```python
from build123d import *

# Parameters (mm, degrees)
SKETCH1_W           = 4
SKETCH1_H           = 70
SKETCH1_H_2         = 60
BOSS_EXTRUDE1_DEPTH = 3
SKETCH1_3_W         = 4
SKETCH1_3_H         = 60
SKETCH1_3_H_2       = 70
BOSS_EXTRUDE2_DEPTH = 70
SKETCH1_4_W         = 4
SKETCH1_4_H         = 70
BOSS_EXTRUDE3_DEPTH = 70
SKETCH5_R           = 4
CUT_EXTRUDE4_DEPTH  = 10
SKETCH6_R           = 2.5
CUT_EXTRUDE5_DEPTH  = 10
SKETCH1_5_W         = 4
SKETCH1_5_H         = 60
BOSS_EXTRUDE4_DEPTH = 80
SKETCH5_2_R         = 4
CUT_EXTRUDE6_DEPTH  = 10
FILLET1_R           = 3
FILLET2_R           = 5
FILLET3_R           = 4
SKETCH7_R           = 2.5
CUT_EXTRUDE7_DEPTH  = 10
SKETCH8_R           = 2.5
CUT_EXTRUDE8_DEPTH  = 10
CUT_EXTRUDE9_REACH  = 132.084
SKETCH9_R           = 3.5
SKETCH26_R          = 2.5
CUT_EXTRUDE11_DEPTH = 10
CUT_EXTRUDE14_DEPTH = 10
CUT_EXTRUDE15_DEPTH = 10
SKETCH28_R          = 1
SKETCH28_R_2        = 4
CUT_EXTRUDE16_DEPTH = 4
SKETCH29_R          = 1
SKETCH29_R_2        = 3.5
CUT_EXTRUDE18_DEPTH = 4
SKETCH31_R          = 5.375
CUT_EXTRUDE19_DEPTH = 10
SKETCH32_W          = 71.641660037
SKETCH32_H          = 79.51751689
CUT_EXTRUDE20_DEPTH = 131.084107183
SKETCH33_W          = 4
SKETCH33_H          = 70
SKETCH33_H_2        = 60
CUT_EXTRUDE21_DEPTH = 71.771465692


with BuildPart() as part:
    # Sketch1 → Boss-Extrude1 (new body)
    # profile 1 of 4: a face of its own
    with BuildSketch(Plane(origin=(0, 0, 0), x_dir=(1, 0, 0), z_dir=(0, 1, 0))):
        Polygon((-50.771305032, 49.212548619), (-50.771305032, 34.212548619), (-46.771305032, 34.212548619), (-46.771305032, -25.787451381), (-50.771305032, -25.787451381), (-50.771305032, -40.787451381), (39.228694968, -40.787451381), (39.228694968, -30.787451381), (35.228694968, -30.787451381), (35.228694968, 39.212548619), (39.228694968, 39.212548619), (39.228694968, 49.212548619), align=None)
        with Locations((-26.271305032, 3.893815937)):
            Rectangle(SKETCH1_W, SKETCH1_H, mode=Mode.SUBTRACT)
    # profile 2 of 4: a face of its own
    with BuildSketch(Plane(origin=(0, 0, 0), x_dir=(1, 0, 0), z_dir=(0, 1, 0))):
        with Locations((37.228694968, 4.212548619)):
            Rectangle(SKETCH1_W, SKETCH1_H)
    # profile 3 of 4: a face of its own
    with BuildSketch(Plane(origin=(0, 0, 0), x_dir=(1, 0, 0), z_dir=(0, 1, 0))):
        with Locations((-48.771305032, 4.212548619)):
            Rectangle(SKETCH1_W, SKETCH1_H_2)
    # profile 4 of 4: a face of its own
    with BuildSketch(Plane(origin=(0, 0, 0), x_dir=(1, 0, 0), z_dir=(0, 1, 0))):
        with Locations((-26.271305032, 3.893815937)):
            Rectangle(SKETCH1_W, SKETCH1_H)
    extrude(amount=BOSS_EXTRUDE1_DEPTH)

    # Sketch1<3> → Boss-Extrude2 (add)
    with BuildSketch(Plane(origin=(0, 0, 0), x_dir=(1, 0, 0), z_dir=(0, 1, 0))):
        with Locations((-48.771305032, 4.212548619)):
            Rectangle(SKETCH1_3_W, SKETCH1_3_H)
        with Locations((37.228694968, 4.212548619)):
            Rectangle(SKETCH1_3_W, SKETCH1_3_H_2)
    extrude(amount=BOSS_EXTRUDE2_DEPTH)

    # Sketch1<4> → Boss-Extrude3 (add)
    with BuildSketch(Plane(origin=(0, 0, 0), x_dir=(1, 0, 0), z_dir=(0, 1, 0))):
        with Locations((-26.271305032, 3.893815937)):
            Rectangle(SKETCH1_4_W, SKETCH1_4_H)
    extrude(amount=BOSS_EXTRUDE3_DEPTH)

    # Sketch5 → Cut-Extrude4 (cut)
    with BuildSketch(Plane.ZY.offset(50.771305032)):
        with Locations((-8.022548619, 60)):
            Circle(SKETCH5_R)
    extrude(amount=-CUT_EXTRUDE4_DEPTH, mode=Mode.SUBTRACT)

    # Sketch6 → Cut-Extrude5 (cut)
    with BuildSketch(Plane(origin=(0, 3, 0), x_dir=(1, 0, 0), z_dir=(0, 1, 0))):
        with Locations(Location((-45.787574368, -35.787451381, 0), (0, 0, 270))):
            Circle(SKETCH6_R)
        with Locations(Location((-45.787574368, 44.212548619, 0), (0, 0, 270))):
            Circle(SKETCH6_R)
        with Locations((43.718511914, 44.212548619)):
            Circle(SKETCH6_R)
        with Locations((43.718511914, -35.787451381)):
            Circle(SKETCH6_R)
    extrude(amount=-CUT_EXTRUDE5_DEPTH, mode=Mode.SUBTRACT)

    # Sketch1<5> → Boss-Extrude4 (add)
    with BuildSketch(Plane(origin=(0, 0, 0), x_dir=(1, 0, 0), z_dir=(0, 1, 0))):
        with Locations((-48.771305032, 4.212548619)):
            Rectangle(SKETCH1_5_W, SKETCH1_5_H)
    extrude(amount=BOSS_EXTRUDE4_DEPTH)

    # Sketch5<2> → Cut-Extrude6 (cut)
    with BuildSketch(Plane.ZY.offset(50.771305032)):
        with Locations((-8.022548619, 60)):
            Circle(SKETCH5_2_R)
    extrude(amount=-CUT_EXTRUDE6_DEPTH, mode=Mode.SUBTRACT)

    # Fillet1
    fillet1_edges = [part.edges().sort_by_distance(p)[0] for p in [
        (-50.771305032, 1.5, 40.787451381),
        (-50.771305032, 1.5, -49.212548619),
        (39.228694968, 1.5, -49.212548619),
        (39.228694968, 1.5, 40.787451381),
    ]]
    fillet(fillet1_edges, radius=FILLET1_R)

    # Fillet2
    fillet2_edges = [part.edges().sort_by_distance(p)[0] for p in [
        (-48.771305032, 80, -34.212548619),
        (-48.771305032, 80, 25.787451381),
        (37.228694968, 70, -39.212548619),
        (37.228694968, 70, 30.787451381),
    ]]
    fillet(fillet2_edges, radius=FILLET2_R)

    # Fillet3
    fillet3_edges = [part.edges().sort_by_distance(p)[0] for p in [
        (-26.271305032, 70, 31.106184063),
        (-26.271305032, 70, -38.893815937),
    ]]
    fillet(fillet3_edges, radius=FILLET3_R)

    # Sketch7 → Cut-Extrude7 (cut)
    with BuildSketch(Plane(origin=(39.228694968, 0, 0), x_dir=(0, 0, -1), z_dir=(1, 0, 0))):
        with Locations((27.482306935, -10)):
            Circle(SKETCH7_R)
    extrude(amount=-CUT_EXTRUDE7_DEPTH, mode=Mode.SUBTRACT)

    # Sketch8 → Cut-Extrude8 (cut)
    with BuildSketch(Plane(origin=(39.228694968, 0, 0), x_dir=(0, 0, -1), z_dir=(1, 0, 0))):
        with Locations((8.02072759, 38.893893193)):
            Circle(SKETCH8_R)
    extrude(amount=-CUT_EXTRUDE8_DEPTH, mode=Mode.SUBTRACT)

    # Cut-Extrude9: up to this face of the body (flat: up to its plane)
    cut_extrude9_end = Plane(part.part.faces().sort_by_distance((-28.271305032, 36.452186393, -3.893815937))[0])
    # Sketch9 → Cut-Extrude9 (cut, up to the picked face)
    with BuildSketch(Plane(origin=(39.228694968, 0, 0), x_dir=(0, 0, -1), z_dir=(1, 0, 0)), mode=Mode.PRIVATE) as cut_extrude9_sk1:
        with Locations((8.02072759, 38.893893193)):
            Circle(SKETCH9_R)
    cut_extrude9_tool1 = split(extrude(cut_extrude9_sk1.sketch, amount=-CUT_EXTRUDE9_REACH, mode=Mode.PRIVATE), bisect_by=cut_extrude9_end, keep=Keep.BOTH, mode=Mode.PRIVATE)
    add(cut_extrude9_tool1.solids().sort_by(Axis((39.228695, 38.893893, -8.020728), (-1, 0, 0)))[0], mode=Mode.SUBTRACT)

    # Sketch26 → Cut-Extrude11 (cut)
    with BuildSketch(Plane(origin=(0, 3, 0), x_dir=(1, 0, 0), z_dir=(0, 1, 0))):
        with Locations(Location((34.228694968, -36.063353705, 0), (0, 0, 270))):
            Circle(SKETCH26_R)
        with Locations(Location((34.228694968, 44.212548619, 0), (0, 0, 270))):
            Circle(SKETCH26_R)
    extrude(amount=-CUT_EXTRUDE11_DEPTH, mode=Mode.SUBTRACT)

    # Sketch27 → Cut-Extrude14 (cut)
    with BuildSketch(Plane(origin=(0, 3, 0), x_dir=(1, 0, 0), z_dir=(0, 1, 0))):
        with BuildLine():
            Line((7.728694968, 3.462548619), (-19.271305032, 3.462548619))
            ThreePointArc((-19.271305032, 3.462548619), (-20.021305032, 4.212548619), (-19.271305032, 4.962548619))
            Line((-19.271305032, 4.962548619), (7.728694968, 4.962548619))
            ThreePointArc((7.728694968, 4.962548619), (8.478694968, 4.212548619), (7.728694968, 3.462548619))
        make_face()
        with BuildLine():
            Line((0.329175915, -7.853794332), (-13.170824085, 15.52889157))
            ThreePointArc((-13.170824085, 15.52889157), (-12.896305032, 16.553410623), (-11.871785979, 16.27889157))
            Line((-11.871785979, 16.27889157), (1.628214021, -7.103794332))
            ThreePointArc((1.628214021, -7.103794332), (1.353694968, -8.128313385), (0.329175915, -7.853794332))
        make_face()
        with BuildLine():
            Line((-13.170824085, -7.103794332), (0.329175915, 16.27889157))
            ThreePointArc((0.329175915, 16.27889157), (1.353694968, 16.553410623), (1.628214021, 15.52889157))
            Line((1.628214021, 15.52889157), (-11.871785979, -7.853794332))
            ThreePointArc((-11.871785979, -7.853794332), (-12.896305032, -8.128313385), (-13.170824085, -7.103794332))
        make_face()
    extrude(amount=-CUT_EXTRUDE14_DEPTH, mode=Mode.SUBTRACT)

    # Sketch27<7> → Cut-Extrude15 (cut)
    with BuildSketch(Plane(origin=(0, 3, 0), x_dir=(1, 0, 0), z_dir=(0, 1, 0))):
        with BuildLine():
            Line((-7.743699741, 2.296260771), (-7.070343138, 3.462548619))
            Line((-7.070343138, 3.462548619), (-8.417056343, 3.462548619))
            ThreePointArc((-8.417056343, 3.462548619), (-8.152874893, 2.837548619), (-7.743699741, 2.296260771))
        make_face()
        with BuildLine():
            Line((-8.417056343, 4.962548619), (-7.070343138, 4.962548619))
            Line((-7.070343138, 4.962548619), (-7.743699741, 6.128836466))
            ThreePointArc((-7.743699741, 6.128836466), (-8.152874893, 5.587548619), (-8.417056343, 4.962548619))
        make_face()
        with BuildLine():
            Line((-5.771305032, 5.712548619), (-5.09794843, 6.878836466))
            ThreePointArc((-5.09794843, 6.878836466), (-5.771305032, 6.962548619), (-6.444661635, 6.878836466))
            Line((-6.444661635, 6.878836466), (-5.771305032, 5.712548619))
        make_face()
        with BuildLine():
            Line((-4.472266927, 4.962548619), (-3.125553721, 4.962548619))
            ThreePointArc((-3.125553721, 4.962548619), (-3.389735172, 5.587548619), (-3.798910324, 6.128836466))
            Line((-3.798910324, 6.128836466), (-4.472266927, 4.962548619))
        make_face()
        with BuildLine():
            ThreePointArc((-3.798910324, 2.296260771), (-3.389735172, 2.837548619), (-3.125553721, 3.462548619))
            Line((-3.125553721, 3.462548619), (-4.472266927, 3.462548619))
            Line((-4.472266927, 3.462548619), (-3.798910324, 2.296260771))
        make_face()
        with BuildLine():
            ThreePointArc((-6.444661635, 1.546260771), (-5.771305032, 1.462548619), (-5.09794843, 1.546260771))
            Line((-5.09794843, 1.546260771), (-5.771305032, 2.712548619))
            Line((-5.771305032, 2.712548619), (-6.444661635, 1.546260771))
        make_face()
    extrude(amount=-CUT_EXTRUDE15_DEPTH, mode=Mode.SUBTRACT)

    # Sketch28 → Cut-Extrude16 (cut)
    # profile 1 of 3: a face of its own
    with BuildSketch(Plane.ZY.offset(50.771305032)):
        with Locations((-2.316893756, 66.434710762)):
            Circle(SKETCH28_R)
    # profile 2 of 3: a face of its own
    with BuildSketch(Plane.ZY.offset(50.771305032)):
        with Locations((-20.69441, 45.708956331)):
            Circle(SKETCH28_R)
    # profile 3 of 3: a face of its own
    with BuildSketch(Plane.ZY.offset(50.771305032)):
        Polygon((-23.458777666, 51.635023443), (-8.531192269, 68.470022529), (0.44747391, 60.508643651), (-14.480111487, 43.673644564), align=None)
        with Locations((-8.022548619, 60)):
            Circle(SKETCH28_R_2, mode=Mode.SUBTRACT)
    extrude(amount=-CUT_EXTRUDE16_DEPTH, mode=Mode.SUBTRACT)

    # Sketch29 → Cut-Extrude18 (cut)
    # profile 1 of 3: a face of its own
    with BuildSketch(Plane(origin=(39.228694968, 0, 0), x_dir=(0, 0, -1), z_dir=(1, 0, 0))):
        with Locations((2.315072727, 45.328603955)):
            Circle(SKETCH29_R)
    # profile 2 of 3: a face of its own
    with BuildSketch(Plane(origin=(39.228694968, 0, 0), x_dir=(0, 0, -1), z_dir=(1, 0, 0))):
        with Locations((20.692588971, 24.602849525)):
            Circle(SKETCH29_R)
    # profile 3 of 3: a face of its own
    with BuildSketch(Plane(origin=(39.228694968, 0, 0), x_dir=(0, 0, -1), z_dir=(1, 0, 0))):
        Polygon((8.529371241, 47.363915722), (23.456956637, 30.528916636), (14.478290458, 22.567537758), (-0.449294939, 39.402536844), align=None)
        with Locations((8.02072759, 38.893893193)):
            Circle(SKETCH29_R_2, mode=Mode.SUBTRACT)
    extrude(amount=-CUT_EXTRUDE18_DEPTH, mode=Mode.SUBTRACT)

    # Sketch31 → Cut-Extrude19 (cut)
    with BuildSketch(Plane(origin=(0, 3, 0), x_dir=(1, 0, 0), z_dir=(0, 1, 0))):
        with Locations((-5.771305032, 4.212548619)):
            Circle(SKETCH31_R)
    extrude(amount=-CUT_EXTRUDE19_DEPTH, mode=Mode.SUBTRACT)

    # Sketch32 → Cut-Extrude20 (cut, through all)
    with BuildSketch(Plane(origin=(39.228694968, 0, 0), x_dir=(0, 0, -1), z_dir=(1, 0, 0))):
        with Locations((4.714645955, 42.758758445)):
            Rectangle(SKETCH32_W, SKETCH32_H)
    extrude(amount=-CUT_EXTRUDE20_DEPTH, mode=Mode.SUBTRACT)

    # Sketch33 → Cut-Extrude21 (cut, through all)
    with BuildSketch(Plane(origin=(0, 3, 0), x_dir=(1, 0, 0), z_dir=(0, 1, 0))):
        with Locations((-26.271305032, 3.893815937)):
            Rectangle(SKETCH33_W, SKETCH33_H)
        with Locations((-48.771305032, 4.212548619)):
            Rectangle(SKETCH33_W, SKETCH33_H_2)
        with Locations((37.228694968, 4.212548619)):
            Rectangle(SKETCH33_W, SKETCH33_H)
    extrude(amount=-CUT_EXTRUDE21_DEPTH, mode=Mode.SUBTRACT)


solid = part.part
```
Geometry: final body of the model. Coordinates: model frame, mm. A direction names the side the tool comes from. Coordinates: 2 decimals unless noted, no trailing zeros. Order: outer loops, then holes, each group sorted by start corner. A loop starts at its lowest first (then second) coordinate and runs counter-clockwise, first axis right, second up. Notation, with made-up numbers: (-27, 6) - (-18, 6) arc R20 cw to (-18, 10) - close; hole circle Ø4 at (36.25, 80). An arc over 180 degrees is marked (long way). Return JSON: item names as keys, results as strings. Group by question number.
1. Cut plane A-A (z = 13). Output: boundary loops of the cut face in (x, y).
2. Pin query (flat end, axial travel): pin 1 (1.5 mm diameter, centred on x = -49.5, y = 1, fed in from -Z); pin 2 (1.5 mm diameter, centred on y = 1, z = -16.5, fed in from +X); pin 3 (3 mm diameter, centred on x = -25.5, z = -7.5, fed in from -Y). Return the tip coordinate at first contact, or that it passes through.
3. Pull-direction query (Z, two-part tool) for faces 4 (the face through (-6, 1, 40.787)), 5 (the face through (-46.745, 1.521, 38.097)), 6 (the face through (39.229, 1, 34)); classes: pulls with the +Z half, pulls with the -Z half, needs draft (parallel to the pull), parting line crosses it, or undercut.
4. Cut plane B-B (y = 2.3). Count the separate pieces of the cut face and the enclosed holes in it, plus the area to 3 significant figures.
5. Material intervals for line 1 along X through (y, z) = (1, -34); line 2 along Z through (x, y) = (6, 1.7); line 3 along X through (y, z) = (1.1, 27.5), sorted ascending. Write a range as [from, to].
6. Set-up query: faces 1 (the face through (-15, 2, -3.463)), 2 (the face through (-49, 2, -34.213)), 3 (the face through (37, 2, 30.787)). Return all of +Z, -Z, +X, -X, +Y, -Y with unobstructed straight access to the full face (end or side cutting, diameter ignored); none if empty.
Resolved:
{
 "1": {"outline": "(-46.77, 0) - (-28.27, 0) - (-28.27, 3) - (-46.77, 3) - close; (-24.27, 0) - (35.23, 0) - (35.23, 3) - (-24.27, 3) - close"},
 "2": {"pin 1": "stops at z = -49.05", "pin 2": "stops at x = 35.23", "pin 3": "stops at y = 0"},
 "3": {"face 4": "pulls with the +Z half", "face 5": "undercut", "face 6": "needs draft"},
 "4": {"separate pieces": "1", "enclosed holes": "6", "area": "7,040 mm²"},
 "5": {"line 1": "x = [-46.77, -28.27], [-24.27, 35.23]", "line 2": "z = [-49.21, -4.96], [-3.46, 40.79]", "line 3": "x = [-50.77, -28.27], [-24.27, 35.23]"},
 "6": {"face 1": "+Y, -Y", "face 2": "-X, +Y, -Y", "face 3": "+X, +Y, -Y"}
}
